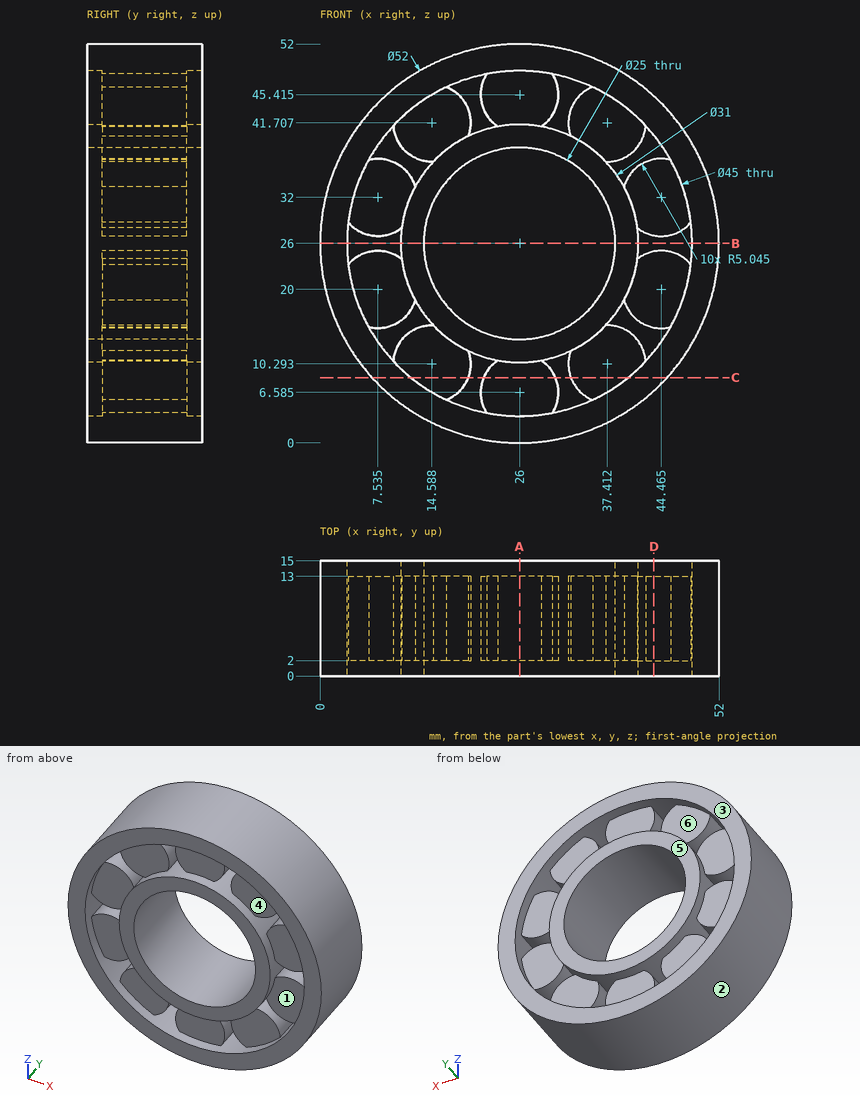
Answer from the drawing. Dimensions are ordinates in mm from the lowest x, y and z of the part. A direction names the side the tool comes from. Give positions to 0.01 mm unless a question says otherwise; leave off trailing zeros. Order: outer loops, then holes, each group sorted by start corner. A loop starts at its lowest first (then second) coordinate and runs counter-clockwise, first axis right, second up.
Item 1: The part is cut by section D-D, the plane x = 43.5. Give the vertices of the cut face in (y, z).
From the geometry:
outline: (0, 6.77) - (15, 6.77) - (15, 11.86) - (0, 11.86) - close; (0, 40.14) - (15, 40.14) - (15, 45.23) - (0, 45.23) - close; (2, 15.05) - (13, 15.05) - (13, 24.95) - (2, 24.95) - close; (2, 27.05) - (13, 27.05) - (13, 36.95) - (2, 36.95) - close
Item 2: Given pin 1 Ø2.5 at (x, z) = (44, 19.5) entering from +Y; pin 2 Ø4.5 at (x, z) = (44.5, 33.5) entering from -Y; pin 3 Ø1 at (x, y) = (15.5, 10) entering from +Z, each flat-ended and moving along its own axis, determine where each tip first touches the part or whether it passes through.
From the geometry:
pin 1: stops at y = 13
pin 2: stops at y = 2
pin 3: stops at z = 50
Item 3: The part is cut by section A-A, the plane x = 26. Give the vertices of the cut face in (y, z), and give its area (3 significant figures).
From the geometry:
outline: (0, 0) - (15, 0) - (15, 3.5) - (13, 3.5) - (13, 10.5) - (15, 10.5) - (15, 13.5) - (0, 13.5) - (0, 10.5) - (2, 10.5) - (2, 3.5) - (0, 3.5) - close; (0, 38.5) - (15, 38.5) - (15, 41.5) - (13, 41.5) - (13, 48.5) - (15, 48.5) - (15, 52) - (0, 52) - (0, 48.5) - (2, 48.5) - (2, 41.5) - (0, 41.5) - close
area: 349 mm2
Item 4: The part is cut by section C-C, the plane z = 8.5. Give the vertices of the cut face in (x, y).
From the geometry:
outline: (6.77, 0) - (11.86, 0) - (11.86, 2) - (19.3, 2) - (19.3, 13) - (11.86, 13) - (11.86, 15) - (6.77, 15) - close; (21.33, 2) - (30.67, 2) - (30.67, 13) - (21.33, 13) - close; (32.7, 2) - (40.14, 2) - (40.14, 0) - (45.23, 0) - (45.23, 15) - (40.14, 15) - (40.14, 13) - (32.7, 13) - close
Item 5: For a pull along Z with two mould halves and no side action, classify the marked faces 1, 2 and 3 as pulls with the +Z half, pulls with the -Z half, needs draft (parallel to the pull), parting line crosses it, or undercut.
From the geometry:
face 1: undercut
face 2: parting line crosses it
face 3: needs draft
Item 6: Which of the six approach directions +Z, -Z, +X, -X, +Y, -Y give full straight-line access (tool end or side, diameter ignored) to the marked faces 4, 5 and 6?
From the geometry:
face 4: -Y
face 5: +Z, -Z, +X, -X, +Y
face 6: +Y
Item 7: Find the intervals of material crossed by probe 1 along Z at (x, y) = (26, 5.5); probe 2 along Z at (x, y) = (8, 2.25) (1 decimal); probe 3 along X at (y, z) = (8.75, 12.5), in increasing order.
From the geometry:
probe 1: z = 0 to 13.5, 38.5 to 52
probe 2: z = 7.2 to 12.5, 15 to 25, 27 to 37, 39.5 to 44.8
probe 3: x = 3.78 to 8, 10.05 to 41.95, 44 to 48.22
Item 8: The part is cut by section B-B, the plane z = 26. Give the vertices of the cut face in (x, y), and give its area (3 significant figures).
From the geometry:
outline: (0, 0) - (3.5, 0) - (3.5, 15) - (0, 15) - close; (10.5, 0) - (13.5, 0) - (13.5, 15) - (10.5, 15) - close; (38.5, 0) - (41.5, 0) - (41.5, 15) - (38.5, 15) - close; (48.5, 0) - (52, 0) - (52, 15) - (48.5, 15) - close
area: 195 mm2
